Geometry: see drawing. Coordinates: mm, zero at the bounding-box minimum. Give positions to 0.01 mm unless a question says otherwise; leave off trailing zeros. Order: outer loops, then holes, each group sorted by start corner. A loop starts at its lowest first (then second) coordinate and runs counter-clockwise, first axis right, second up. Notation, with made-up numbers: (44, 83) - (56, 83) arc R17 ccw to (56, 98) - close; hole circle Ø2 at (86, 61.5). An arc over 180 degrees is marked (long way). One line per item, written item: value.
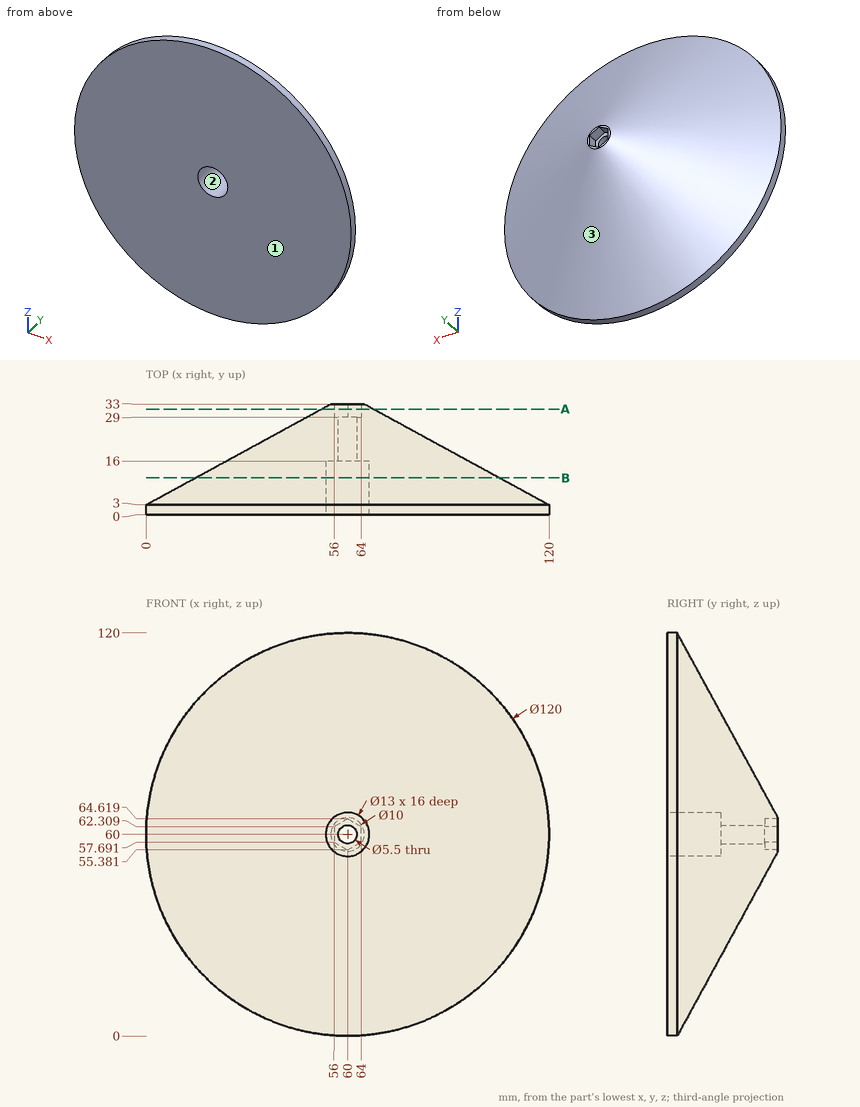
1) Section B-B, the plane y = 11. Return loops of the section in (x, z), then the cut area to 3 significant figures.
Answers below:
outline: circle Ø90.67 at (60, 60); hole circle Ø13 at (60, 60)
area: 6,320 mm^2
2) Mould query, pull axis X, two halves, no side actions, for the marked faces 1, 2 and 3. Classes: released by +X, released by -X, zero draft, split by the parting line, or undercut.
Answers below:
face 1: zero draft
face 2: undercut
face 3: split by the parting line
3) Material intervals for line 1 along Z through (x, y) = (60, 11) (1 decimal); line 2 along Y through (x, z) = (46.5, 13) (1 decimal); line 3 along Y through (x, z) = (61, 18.5) (1 decimal), sorted ascending.
Answers below:
line 1: 14.7 to 53.5, 66.5 to 105.3
line 2: 0 to 9.1
line 3: 0 to 13.1
4) First-contact query: pin 1 (10.5 mm diameter, centred on x = 60, z = 60, fed in from -Y); pin 2 (2 mm diameter, centred on y = 32, z = 60, fed in from -X) (1 decimal); pin 3 (2.5 mm diameter, centred on x = 58, z = 61.5, fed in from +Y); pin 4 (5 mm diameter, centred on y = 27.5, z = 85.5, fed in from -X). Flat tips, straight axial feed; report the tip coordinate or a pass-through.
Answers below:
pin 1: y = 16
pin 2: x = 51.3
pin 3: y = 29
pin 4: through
5) Section A-A, the plane y = 31.5. Return loops of the section in (x, z), then the cut area to 3 significant figures.
Answers below:
outline: circle Ø15.5 at (60, 60); hole (56, 57.69) - (60, 55.38) - (64, 57.69) - (64, 62.31) - (60, 64.62) - (56, 62.31) - close
area: 133 mm^2
